Check sheet for the modelled part. Datum: model origin and axes. Units: mm. A direction names the side the tool comes from. Coordinates: 2 decimals unless noted, no trailing zeros. Loops run counter-clockwise (first coordinate to the right, second up) from the corner with the lowest first, then second, coordinate; pieces in that order, holes last. Notation, with made-up numbers: (78.25, 7) - (112.25, 7) arc R23 ccw to (112.25, 41) - close; hole circle Ø6 at (74, -38.75). An arc over 180 degrees is marked (long way). Answer as a JSON object with one key per item and string values. Group by question number.
from build123d import *

# Parameters (mm, degrees)
F0_R     = 11.12
F0_R_2   = 5.44
F1_DEPTH = 23.48
F3_R     = 10.25
F3_R_2   = 5.44
F4_DEPTH = 1.08
F6_R     = 11.46
F6_R_2   = 5.44
F7_DEPTH = 3
F8_SIZE  = 1.28
F9_SIZE  = 1.28
F10_SIZE = 1.28


with BuildPart() as f1:
    # F0 (on Top) → F1 (new body)
    with BuildSketch(Plane.XY):
        Circle(F0_R)
        Circle(F0_R_2, mode=Mode.SUBTRACT)
    extrude(amount=F1_DEPTH)

    # F3 (on offset) → F4 (join)
    with BuildSketch(Plane.XY.offset(23.48)):
        Circle(F3_R)
        Circle(F3_R_2, mode=Mode.SUBTRACT)
    extrude(amount=F4_DEPTH)

    # F6 (on offset) → F7 (join)
    with BuildSketch(Plane.XY.offset(24.56)):
        Circle(F6_R)
        Circle(F6_R_2, mode=Mode.SUBTRACT)
    extrude(amount=F7_DEPTH)

    # F8
    f8_edges = [f1.edges().sort_by_distance(p)[0] for p in [
        (-11.12, 0, 0),
    ]]
    chamfer(f8_edges, length=F8_SIZE)

    # F9
    f9_edges = [f1.edges().sort_by_distance(p)[0] for p in [
        (-5.44, 0, 0),
    ]]
    chamfer(f9_edges, length=F9_SIZE)

    # F10
    f10_edges = [f1.edges().sort_by_distance(p)[0] for p in [
        (-5.44, 0, 27.56),
    ]]
    chamfer(f10_edges, length=F10_SIZE)


solid = f1.part
1. Sectioned sample at C-C on z = 14. Record the cut outline in (x, y), plus the area to 4 significant figures.
2. Sectioned sample at A-A on y = 0. Record the cut outline in (x, z).
3. Material ranges on line 1 (Y direction, x = 0, z = 14.25); line 2 (Z direction, x = 9, y = -5); line 3 (Y direction, x = -3.5, z = 18.25), recorded low to high.
4. Access from +Z, -Z, +X, -X, +Y, -Y to the whole of each face (thin tool, end or side, straight path). Record for faces 4 (the face through (4, -6, 0)), 5 (the face through (-8.8, -6.8, 12.2)), 6 (the face through (-2.222, -10.006, 24.012)).
5. Gauge pin test, flat ends, axial feed: pin 1 (10 mm diameter, centred on x = 5, y = 3.5, fed in from +Z); pin 2 (12 mm diameter, centred on y = -9, z = 24.5, fed in from +X); pin 3 (4 mm diameter, centred on x = -8.5, z = 16, fed in from +Y); pin 4 (8 mm diameter, centred on x = 5, z = 4.5, fed in from +Y). Record the tip position at first contact, or that the pin passes through.
6. Release check for a two-part mould opening along Y. For faces 1 (the face through (-11.45, 0.5, 26.04)), 2 (the face through (5.2, 1.6, 13.6)), 3 (the face through (3, -10, 23.48)) record: released by +Y, released by -Y, zero draft, split by the parting line, or undercut.
Answers follow:
{
 "1": {"outline": "circle Ø22.24 at (0, 0); hole circle Ø10.88 at (0, 0)", "area": "295.5 mm^2"},
 "2": {"outline": "(-11.46, 24.56) - (-10.25, 24.56) - (-10.25, 23.48) - (-11.12, 23.48) - (-11.12, 1.28) - (-9.84, 0) - (-6.72, 0) - (-5.44, 1.28) - (-5.44, 26.28) - (-6.72, 27.56) - (-11.46, 27.56) - close; (5.44, 1.28) - (6.72, 0) - (9.84, 0) - (11.12, 1.28) - (11.12, 23.48) - (10.25, 23.48) - (10.25, 24.56) - (11.46, 24.56) - (11.46, 27.56) - (6.72, 27.56) - (5.44, 26.28) - close"},
 "3": {"line 1": "y = -11.12 to -5.44, 5.44 to 11.12", "line 2": "z = 0.46 to 23.48, 24.56 to 27.56", "line 3": "y = -10.55 to -4.16, 4.16 to 10.55"},
 "4": {"face 4": "-Z, +X, -X, +Y, -Y", "face 5": "-Z", "face 6": "none"},
 "5": {"pin 1": "stops at z = 27.56", "pin 2": "stops at x = 11.06", "pin 3": "stops at y = 9.02", "pin 4": "stops at y = 11.07"},
 "6": {"face 1": "split by the parting line", "face 2": "undercut", "face 3": "zero draft"}
}
